from build123d import *

# Parameters (mm, degrees)
F0_W     = 74
F0_H     = 74
F1_DEPTH = 900
F2_W     = 67
F2_H     = 74
F3_DEPTH = 10
F4_R     = 5
F5_DEPTH = 25


# Not quite as in the source:
# - a pattern or mirror of a feature is missing from the dataset's text; its kind, count and spacing are read off the source's solid


with BuildPart() as f1:
    # F0 (on Front) → F1 (new body)
    with BuildSketch(Plane.XZ):
        with BuildLine():
            ThreePointArc((40, 35), (38.5355339059, 38.5355339059), (35, 40))
            Line((35, 40), (-35, 40))
            ThreePointArc((-35, 40), (-38.5355339059, 38.5355339059), (-40, 35))
            Line((-40, 35), (-40, -35))
            ThreePointArc((-40, -35), (-38.5355339059, -38.5355339059), (-35, -40))
            Line((-35, -40), (35, -40))
            ThreePointArc((35, -40), (38.5355339059, -38.5355339059), (40, -35))
            Line((40, -35), (40, 35))
        make_face()
        Rectangle(F0_W, F0_H, mode=Mode.SUBTRACT)
    extrude(amount=F1_DEPTH)

    # F2 (on face) → F3 (join)
    with BuildSketch(Plane.XZ.offset(900)):
        with Locations((3.5, 0)):
            Rectangle(F2_W, F2_H)
        with BuildLine():
            Line((-30, -37), (-30, -40))
            Line((-30, -40), (35, -40))
            ThreePointArc((35, -40), (38.5355339059, -38.5355339059), (40, -35))
            Line((40, -35), (40, 35))
            ThreePointArc((40, 35), (38.5355339059, 38.5355339059), (35, 40))
            Line((35, 40), (-30, 40))
            Line((-30, 40), (-30, 37))
            Line((-30, 37), (37, 37))
            Line((37, 37), (37, -37))
            Line((37, -37), (-30, -37))
        make_face()
        with BuildLine():
            ThreePointArc((40, -35), (38.5355339059, -38.5355339059), (35, -40))
            Line((35, -40), (40, -40))
            Line((40, -40), (40, -35))
        make_face()
        with BuildLine():
            ThreePointArc((35, 40), (38.5355339059, 38.5355339059), (40, 35))
            Line((40, 35), (40, 60))
            Line((40, 60), (-30, 60))
            Line((-30, 60), (-30, 40))
            Line((-30, 40), (35, 40))
        make_face()
    f3 = extrude(amount=F3_DEPTH)

    # F3_copies: F3 across plane
    add(f3.mirror(Plane.ZX.offset(-450)))

    # F4 (on face) → F5 (cut)
    with BuildSketch(Plane(origin=(0, -900, 0), x_dir=(-1, 0, 0), z_dir=(0, 1, 0))):
        with Locations((-25, 50)):
            Circle(F4_R)
        with Locations((15, 50)):
            Circle(F4_R)
        with Locations((15, 25)):
            Circle(F4_R)
        with Locations((-25, 25)):
            Circle(F4_R)
        with Locations((-25, -25)):
            Circle(F4_R)
        with Locations((15, -25)):
            Circle(F4_R)
    f5 = extrude(amount=-F5_DEPTH, mode=Mode.SUBTRACT)

    # F5_copies: F5 across plane
    add(f5.mirror(Plane.ZX.offset(-450)), mode=Mode.SUBTRACT)


solid = f1.part
Model file for the job. Use its own axes, mm. A direction names the side the tool comes from. Round coordinates to 2 decimals unless told otherwise and drop trailing zeros. Loops run counter-clockwise (first coordinate to the right, second up) from the corner with the lowest first, then second, coordinate; pieces in that order, holes last. Notation, with made-up numbers: (-38.5, 6) -> (-10.5, 6) arc R26 ccw to (-10.5, 40) -> close; hole circle Ø8 at (71, 61.5). An arc over 180 degrees is marked (long way). Answer as CSV lines item,"result". Start each with the question number.
1) Probe line 1 along X through (y, z) = (5.5, 50); line 2 along Z through (x, y) = (-15, -907.5); line 3 along Y through (x, z) = (-2.5, -21). List the from-to ranges inside material, lowest first.
2) Slice it at A-A (z = 0.5). List the corners of the cut face in (x, y), plus the area to 3 significant figures.
3) Pin check, flat tips, straight feed: P1, Ø3, axis at y = -902.5, z = 16, coming from the -X side; P2, Ø8, axis at x = -15, z = -25, coming from the +Y side; P3, Ø1, axis at y = -537, z = 38.5, coming from the -X side; P4, Ø21, axis at x = -3.5, y = -664, coming from the +Z side. Stop position of each tip, or through.
4) Slice it at B-B (y = -258.5). List the corners of the cut face in (x, z).
5) Tool access for faces 5 (the face through (-37, -444, -1)), 6 (the face through (0, -444, 40)), 7 (the face through (-1, -444, 37)): list every direction of +Z, -Z, +X, -X, +Y, -Y with a clear straight run to the whole face (end or side of a thin tool).
6) Mould opens along Y. For faces 1 (the face through (40, -456, 9)), 2 (the face through (5, -910, 11)), 3 (the face through (3, -900, 1)), 4 (the face through (3, 0, 1)) say: +Y half, -Y half, draft (parallel to the pull), parting line (faces both ways), or undercut.
Filled in:
1,line 1,"x = -30 to -20, -10 to 20, 30 to 40"
1,line 2,"z = -40 to -30, -20 to 20, 30 to 45, 55 to 60"
1,line 3,"y = -910 to -900, 0 to 10"
2,outline,"(-40, -900) -> (-37, -900) -> (-37, 0) -> (-40, 0) -> close; (-30, -910) -> (40, -910) -> (40, 10) -> (-30, 10) -> (-30, 0) -> (37, 0) -> (37, -900) -> (-30, -900) -> close"
2,area,"6,800 mm2"
3,P1,"stops at x = -30"
3,P2,"passes through"
3,P3,"stops at x = -39"
3,P4,"stops at z = 40"
4,outline,"(-40, -35) arc R5 ccw to (-35, -40) -> (35, -40) arc R5 ccw to (40, -35) -> (40, 35) arc R5 ccw to (35, 40) -> (-35, 40) arc R5 ccw to (-40, 35) -> close; hole (-37, -37) -> (37, -37) -> (37, 37) -> (-37, 37) -> close"
5,face 5,"+Y, -Y"
5,face 6,"+Z, +X, -X"
5,face 7,"none"
6,face 1,"draft"
6,face 2,"-Y half"
6,face 3,"undercut"
6,face 4,"undercut"
